Work out the finished part from the listing and answer in its coordinate system (mm). Face numbers are marked on the shaded views. A direction names the side the tool comes from. Give positions to 0.01 mm unless a question says otherwise; leave off trailing zeros. Loops run counter-clockwise (first coordinate to the right, second up) from the corner with the lowest first, then second, coordinate; pieces in that order, holes last. Notation, with made-up numbers: (27.25, 74.5) - (84.25, 74.5) arc R26 ccw to (84.25, 101.5) - close; hole circle Ø11 at (19.25, 32). An arc over 180 degrees is marked (long way). Use CSV: the item, a comma, the result in double quotes.
from build123d import *

# Parameters (mm, degrees)
SKETCH1_W               = 22.054431489
SKETCH1_H               = 12.5
BOSS_EXTRUDE1_DEPTH     = 34
CUT_EXTRUDE1_DEPTH      = 10
CUT_EXTRUDE1_DEPTH_BACK = 15
SKETCH2_R               = 1.5
FILLET3_R               = 2
SKETCH5_R               = 1.5
CUT_EXTRUDE4_DEPTH      = 52.610795679
SKETCH16_W              = 22.066089364
SKETCH16_H              = 2.745994046
SKETCH16_H_2            = 2.696035541
CUT_EXTRUDE6_DEPTH      = 14.5
FILLET4_R               = 1
SKETCH17_W              = 18.252824183
SKETCH17_H              = 2.745994046
SKETCH17_H_2            = 2.696035541
CUT_EXTRUDE7_DEPTH      = 5
SKETCH18_W              = 24.333833062
SKETCH18_H              = 0.605314718
SKETCH18_H_2            = 0.725933663
CUT_EXTRUDE8_DEPTH      = 20


with BuildPart() as part:
    # Sketch1 → Boss-Extrude1 (new body)
    with BuildSketch(Plane.XY):
        with Locations((-13.228930986, -24.070183414)):
            Rectangle(SKETCH1_W, SKETCH1_H)
    extrude(amount=BOSS_EXTRUDE1_DEPTH)

    # Sketch2 → Cut-Extrude1 (cut, two sides: drawn at the far end of the back side and taken through both)
    with BuildSketch(Plane.XZ.offset(30.320183414).offset(-CUT_EXTRUDE1_DEPTH_BACK)):
        with Locations(Location((-13.228930986, 6.5, 0), (0, 0, 90))):
            Circle(SKETCH2_R)
        with Locations(Location((-13.228930986, 29, 0), (0, 0, 90))):
            Circle(SKETCH2_R)
        with BuildLine():
            Line((-4.315096089, 25.086165103), (-2.201715242, 25.086165103))
            add(Edge.make_bspline(
                [(-24.256146731, 25.458595261), (-35.656041951, 36.540332573), (-13.006901701, 52.285060009), (9.32231541, 36.338450422), (-2.201715242, 25.086165103)],
                knots=[0, 0, 0, 0, 0.496841919, 1, 1, 1, 1], degree=3))
            add(Edge.make_bspline(
                [(-13.228930986, 34), (-19.086447972, 37.422293362), (-24.885707195, 30.868976401), (-24.256146731, 25.458595261)],
                knots=[0, 0, 0, 0, 1, 1, 1, 1], degree=3))
            ThreePointArc((-13.228930986, 34), (-6.925897884, 31.389198205), (-4.315096089, 25.086165103))
        make_face()
        with BuildLine():
            Line((-4.478930986, 8.75), (-2.201715242, 8.75))
            add(Edge.make_bspline(
                [(-2.201715242, 8.75), (5.39210746, 3.880294823), (-0.777052631, -4.523329032), (-17.174300591, -10.623347238), (-34.821400648, -0.026005424), (-24.256146731, 8.75)],
                knots=[0, 0, 0, 0, 0.283272691, 0.504244858, 1, 1, 1, 1], degree=3))
            add(Edge.make_bspline(
                [(-23.490579314, 0), (-24.966512963, 4.237786421), (-24.256146731, 8.75)],
                knots=[0, 0, 0, 1, 1, 1], degree=2))
            Line((-23.490579314, 0), (-13.228930986, 0))
            ThreePointArc((-13.228930986, 0), (-7.041746651, 2.562815665), (-4.478930986, 8.75))
        make_face()
    extrude(amount=CUT_EXTRUDE1_DEPTH + CUT_EXTRUDE1_DEPTH_BACK, mode=Mode.SUBTRACT)

    # Fillet3
    # the kernel refuses this fillet: 2 mm, written as the material it takes off along each edge
    with BuildSketch(Plane(origin=(-24.256146731, -17.820183414, -1.998495188), x_dir=(1, 0, 0), z_dir=(0, 0, 1))) as fillet3_piece_1:
        with BuildLine():
            CenterArc((FILLET3_R, -FILLET3_R), FILLET3_R, 90, 90)
            Line((0, -FILLET3_R), (0, 0))
            Line((0, 0), (FILLET3_R, 0))
        make_face()
    extrude(amount=34.125242274, mode=Mode.SUBTRACT)
    with BuildSketch(Plane(origin=(-24.256146731, -30.320183414, -1.998495188), x_dir=(1, 0, 0), z_dir=(0, 0, 1))) as fillet3_piece_2:
        with BuildLine():
            CenterArc((FILLET3_R, FILLET3_R), FILLET3_R, 180, 90)
            Line((0, FILLET3_R), (0, 0))
            Line((0, 0), (FILLET3_R, 0))
        make_face()
    extrude(amount=34.125242274, mode=Mode.SUBTRACT)
    with BuildSketch(Plane(origin=(-24.256146731, -17.374523396, 3.001504812), x_dir=(0.1667681859257429, 1.4874647964432132e-15, -0.9859961319209304), z_dir=(0, -1, 0))) as fillet3_piece_3:
        with BuildLine():
            CenterArc((0.168096911, 1.999974157), FILLET3_R, 260.400032587, 9.891234523)
            Line((-0.165439461, 0.027981894), (0, 0))
            ThreePointArc((0, 0), (0.089132004, -0.000226606), (0.178264007, 0))
        make_face()
    extrude(amount=13.331280444, mode=Mode.SUBTRACT)
    with BuildSketch(Plane(origin=(-24.256146731, -17.482274803, 27.126747086), x_dir=(0.11756979569322837, -1.02728794699617e-15, 0.9930646218351818), z_dir=(0, -1, 0))) as fillet3_piece_4:
        with BuildLine():
            CenterArc((0.118560979, -1.999931088), FILLET3_R, 89.524368939, 7.227500304)
            Line((-0.116578613, -0.013801845), (0, 0))
            ThreePointArc((0, 0), (0.067581725, 0.000281106), (0.135163444, 0))
        make_face()
    extrude(amount=13.131401648, mode=Mode.SUBTRACT)

    # Sketch5 → Cut-Extrude4 (cut, through all)
    with BuildSketch(Plane.XY):
        with Locations((-18.011106811, -24.070183414)):
            Circle(SKETCH5_R)
        with Locations(Location((-8.446755162, -24.070183414, 0), (0, 0, 180))):
            Circle(SKETCH5_R)
    extrude(amount=CUT_EXTRUDE4_DEPTH, mode=Mode.SUBTRACT)

    # Sketch16 → Cut-Extrude6 (cut)
    with BuildSketch(Plane.XY.offset(38)):
        with Locations((-13.228930985, -20.307980077)):
            Rectangle(SKETCH16_W, SKETCH16_H)
        with Locations((-13.228930985, -28.109934669)):
            Rectangle(SKETCH16_W, SKETCH16_H_2)
    extrude(amount=-CUT_EXTRUDE6_DEPTH, mode=Mode.SUBTRACT)

    # Fillet4
    fillet4_edges = [part.edges().sort_by_distance(p)[0] for p in [
        (-2.201715242, -29.889067926, 25.086165103),
    ]]
    fillet(fillet4_edges, radius=FILLET4_R)

    # Sketch17 → Cut-Extrude7 (cut)
    with BuildSketch(Plane.XY.offset(23.5)):
        with Locations((-13.345007216, -20.307980077)):
            Rectangle(SKETCH17_W, SKETCH17_H)
        with Locations((-13.345007216, -28.109934669)):
            Rectangle(SKETCH17_W, SKETCH17_H_2)
    extrude(amount=-CUT_EXTRUDE7_DEPTH, mode=Mode.SUBTRACT)

    # Sketch18 → Cut-Extrude8 (cut)
    with BuildSketch(Plane.XY):
        with Locations((-12.791033736, -17.704302546)):
            Rectangle(SKETCH18_W, SKETCH18_H)
        with Locations((-12.791033736, -30.407371646)):
            Rectangle(SKETCH18_W, SKETCH18_H_2)
    extrude(amount=CUT_EXTRUDE8_DEPTH, mode=Mode.SUBTRACT)


solid = part.part
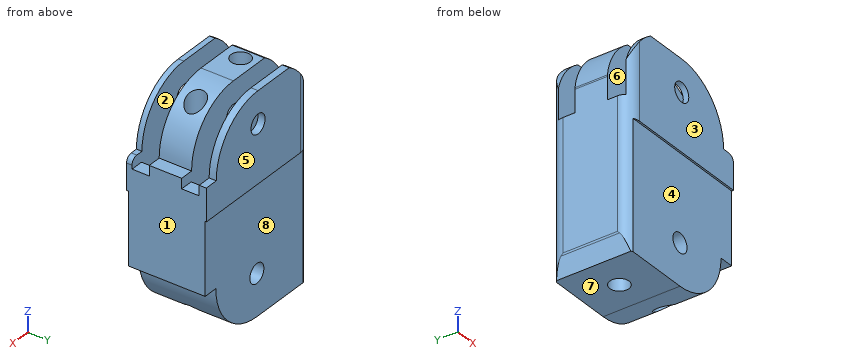
Item 1: A cutting plane is placed at B-B on z = 6.5. Determine the outline of the cut face in (x, y), and give its area (3 significant figures).
Determined:
outline,"(-24.26, -28.32) arc R2 ccw to (-23.27, -30.04) - (-14.73, -30.04) - (-14.73, -18.01) - (-23.1, -18.01) arc R2 ccw to (-24.26, -19.82) - close; (-11.73, -30.04) - (-4.77, -30.04) - (-4.77, -18.01) - (-11.73, -18.01) - close; hole circle Ø3 at (-18.01, -24.07); hole circle Ø3 at (-8.45, -24.07)"
area,"183 mm²"
Item 2: The mould has two halves that part along Y. Classify the marked faces 1, 2 and 3: pulls with the +Y half, pulls with the -Y half, needs draft (parallel to the pull), parting line crosses it, or undercut.
Determined:
face 1,"needs draft"
face 2,"undercut"
face 3,"pulls with the -Y half"
Item 3: A cutting plane is placed at C-C on x = -8.75. Determine the outline of the cut face in (y, z).
Determined:
outline,"(-30.32, 20) - (-30.04, 20) - (-30.04, 1.23) - (-25.54, 1.23) - (-25.54, 32.79) - (-26.76, 32.79) - (-26.76, 18.5) - (-29.46, 18.5) - (-29.46, 32.79) - (-30.32, 32.79) - close; (-22.6, 1.23) - (-18.01, 1.23) - (-18.01, 20) - (-17.82, 20) - (-17.82, 32.79) - (-18.93, 32.79) - (-18.93, 18.5) - (-21.68, 18.5) - (-21.68, 32.79) - (-22.6, 32.79) - close"
Item 4: Given P1, Ø6, axis at x = -16, z = 9, coming from the +Y side; P2, Ø1.4, axis at x = -23.5, y = -20, coming from the +Z side; P3, Ø2, axis at x = -9.5, y = -28, coming from the +Z side, each flat-ended and moving along its own axis, determine where each tip first touches the part or whether it passes through.
Determined:
P1,"stops at y = -18.01"
P2,"stops at z = 23.5"
P3,"stops at z = 18.5"
Item 5: For the marked faces 4, 5, 6, 7 and 8, determine the directions among +Z, -Z, +X, -X, +Y, -Y from which every point of the face is accessible in a straight line to the end or side of a thin tool.
Determined:
face 4,"-Z, +X, -X, -Y"
face 5,"+Z, -Z, +X, -X, +Y"
face 6,"+Z"
face 7,"-Z, +X, -X, +Y, -Y"
face 8,"-Z, +X, -X, +Y"
Item 6: Find the intervals of material crossed by line 1 (X direction, y = -24.25, z = 26.5); line 2 (Y direction, x = -18.5, z = 32.5); line 3 (X direction, y = -22.9, z = 29), in increasing order.
Determined:
line 1,"x = -24.26 to -19.5, -16.52 to -9.94, -6.96 to -4.43"
line 2,"y = -30.32 to -29.46, -26.76 to -25.49, -22.65 to -21.68, -18.93 to -17.82"
line 3,"x = -23.83 to -18.95, -17.07 to -14.73, -11.73 to -9.39, -7.51 to -5.22"
Item 7: A cutting plane is placed at A-A on x = -12.5. State how many separate pieces and enclosed holes the cut face has, and give its area (3 significant figures).
Determined:
separate pieces,"5"
enclosed holes,"0"
area,"281 mm²"
